Here's how the part is built. I have some questions about the finished solid (model axes, mm). A direction names the side the tool comes from. Round coordinates to 2 decimals unless told otherwise and drop trailing zeros. Write each loop counter-clockwise with the first axis right and the second up, starting at its lowest first coordinate (ties: lowest second). Pieces come first, ordered by that corner, then holes. Notation, with made-up numbers: (-29, 3.5) - (21, 3.5) arc R6 cw to (21, 10.5) - close; hole circle Ø5 at (34, -24.5). An arc over 180 degrees is marked (long way). One line per question, with ' | ' between items. Start each with the question number.
(1) Imagine slicing it at C-C (z = 3). Write out the boundary of the cut face in (x, y).
(2) Imagine slicing it at A-A (x = 0). Write out the boundary of the cut face in (y, z).
(3) Imagine slicing it at D-D (z = 11). Write out the boundary of the cut face in (x, y), plus the area to 3 significant figures.
(4) For faces 1 (the cylindrical face through (0.26, 26.71, 4.44)), 2 (the flat face through (6.25, -13, 11)), 3 (the flat face through (0, -9.689, 11)), which set-ups out of +Z, -Z, +X, -X, +Y, -Y let a thin tool reach every point of the face, with its end or its side?
(5) If I drill on L1, parallel to Y at x = 0, z = 4.5; L2, parallel to Z at x = 8.5, y = -11.5; L3, parallel to X at y = 14.5, z = 8, over which ranges is the centre line in solid material (lowest first)?
(6) Will these pins go through, and if not, where does the flat tip stop? pin 1 (2 mm diameter, centred on x = 9.5, y = 21.5, fed in from +Z); pin 2 (2.5 mm diameter, centred on x = 0, z = 12.5, fed in from +Y); pin 3 (5 mm diameter, centred on x = -5.5, z = 10.5, fed in from +Y); pin 4 (9 mm diameter, centred on x = 0, y = 11.21, fed in from -Z).
(7) Imagine slicing it at B-B (y = 8). Write out the boundary of the cut face in (x, z).
(8) Thinking about a two-plate mould opening in X: for faces 4 (the flat face through (14.5, 0, 4)), 5 (the cylindrical face through (-5.64, 16.38, 4.44)), 6 (the flat face through (0, 0, 0)), 7 (the flat face through (-6.25, -13, 11)), which applies, pulls with the +X half, pulls with the -X half, needs draft (parallel to the pull), parting line crosses it, or undercut?
from build123d import *

# Parameters (mm, degrees)
SKETCH1_R           = 7.65
BOSS_EXTRUDE1_DEPTH = 9
SKETCH2_W           = 12.5
SKETCH2_H           = 7
BOSS_EXTRUDE2_DEPTH = 5


with BuildPart() as part:
    # Sketch1 → Boss-Extrude1 (new body)
    with BuildSketch(Plane.XY):
        with BuildLine():
            Line((-14.5, -16.688612788), (14.5, -16.688612788))
            Line((14.5, -16.688612788), (14.5, 16.688612788))
            ThreePointArc((14.5, 16.688612788), (0, 26.711387212), (-14.5, 16.688612788))
            Line((-14.5, 16.688612788), (-14.5, -16.688612788))
        make_face()
        with Locations((0, 11.211387212)):
            Circle(SKETCH1_R, mode=Mode.SUBTRACT)
    extrude(amount=BOSS_EXTRUDE1_DEPTH)

    # Sketch2 → Boss-Extrude2 (add)
    with BuildSketch(Plane.XY.offset(9)):
        with Locations((0, -13.188612788)):
            Rectangle(SKETCH2_W, SKETCH2_H)
    extrude(amount=BOSS_EXTRUDE2_DEPTH)


solid = part.part
Check sheet entries:
1) outline: (-14.5, -16.69) - (14.5, -16.69) - (14.5, 16.69) arc R15.5 ccw to (-14.5, 16.69) - close; hole circle Ø15.3 at (0, 11.21)
2) outline: (-16.69, 0) - (3.56, 0) - (3.56, 9) - (-9.69, 9) - (-9.69, 14) - (-16.69, 14) - close; (18.86, 0) - (26.71, 0) - (26.71, 9) - (18.86, 9) - close
3) outline: (-6.25, -16.69) - (6.25, -16.69) - (6.25, -9.69) - (-6.25, -9.69) - close | area: 87.5 mm^2
4) face 1: +Z, -Z, +Y | face 2: +Z, +X, +Y, -Y | face 3: +Z, +X, -X, +Y
5) L1: -16.69 to 3.56, 18.86 to 26.71 | L2: 0 to 9 | L3: -14.5 to -6.91, 6.91 to 14.5
6) pin 1: z = 9 | pin 2: y = -9.69 | pin 3: y = 26.31 | pin 4: through
7) outline: (-14.5, 0) - (-6.94, 0) - (-6.94, 9) - (-14.5, 9) - close; (6.94, 0) - (14.5, 0) - (14.5, 9) - (6.94, 9) - close
8) face 4: pulls with the +X half | face 5: undercut | face 6: needs draft | face 7: pulls with the -X half
